Input: part model. Units: mm. Frame: model coordinates. A direction names the side the tool comes from. Round coordinates to 2 decimals unless told otherwise and drop trailing zeros. Loops run counter-clockwise (first coordinate to the right, second up) from the corner with the lowest first, then second, coordinate; pieces in that order, holes last. Notation, with made-up numbers: (46.25, -37.75) -> (67.25, -37.75) arc R9 ccw to (67.25, -27.75) -> close; hole circle Ø1 at (-37.75, -31). An arc over 180 degrees is marked (long way). Answer as a JSON object with one key per item and string values.
```python
from build123d import *

# Parameters (mm, degrees)
F0_R     = 3.175
F1_DEPTH = 25.4
F0_R_2   = 38.1
F2_DEPTH = 12.7
F3_W     = 16.933164
F3_H     = 50.8
F3_W_2   = 16.933333164
F4_DEPTH = 50.8
F5_R     = 25.39999
F6_R     = 3.175
F7_DEPTH = 103.2441
F8_DEPTH = 120.64677


# Not quite as in the source:
# - a fillet or chamfer is up to 0.001 mm smaller than in the source, because OpenCascade refuses the exact size


with BuildPart() as f1:
    # F0 (on Top) → F1 (new body)
    with BuildSketch(Plane.XY):
        Circle(F0_R)
    extrude(amount=-F1_DEPTH)

    # F0 (on Top) → F2 (join)
    with BuildSketch(Plane.XY):
        Circle(F0_R_2)
        Circle(F0_R, mode=Mode.SUBTRACT)
        Circle(F0_R)
    extrude(amount=F2_DEPTH)

    # F3 (on face) → F4 (join)
    with BuildSketch(Plane.XY.offset(12.7)):
        with Locations((16.933418, 0)):
            Rectangle(F3_W, F3_H)
        with Locations((-16.933333418, 0)):
            Rectangle(F3_W_2, F3_H)
    extrude(amount=F4_DEPTH)

    # F5 (radius 25.4 in the source; OpenCascade refuses exactly that, so slightly less here)
    f5_edges = [f1.edges().sort_by_distance(p)[0] for p in [
        (16.933418, -25.4, 63.5),
        (16.933418, 25.4, 63.5),
        (-16.933333, 25.4, 63.5),
        (-16.933333, -25.4, 63.5),
    ]]
    fillet(f5_edges, radius=F5_R)

    # F6 (on face) → F7 (cut)
    with BuildSketch(Plane(origin=(-25.4, 0, 0), x_dir=(0, -1, 0), z_dir=(-1, 0, 0))):
        with Locations((0, 38.1)):
            Circle(F6_R)
    extrude(amount=-F7_DEPTH, mode=Mode.SUBTRACT)

    # F8 (cut): a face of the model
    f8_faces = [f1.faces().sort_by_distance(p)[0] for p in [
        (0, 0, -25.4),
    ]]
    extrude(f8_faces, amount=-F8_DEPTH, mode=Mode.SUBTRACT)


solid = f1.part
```
1) Ray query, probe 1 along X at (y, z) = (16, 14); probe 2 along Z at (x, y) = (13.25, 0) (3 decimals); probe 3 along Y at (x, z) = (0, 4.25) (3 decimals). Return the intervals inside material, ascending.
Output:
{"probe 1": "x = -25.4 to -8.47, 8.47 to 25.4", "probe 2": "z = 0 to 34.925, 41.275 to 63.5", "probe 3": "y = -38.1 to -3.175, 3.175 to 38.1"}
2) Section B-B, the plane z = 54. Output: boundary loops of the cut face in (x, y).
Output:
{"outline": "(-25.4, -19.81) -> (-8.47, -19.81) -> (-8.47, 19.81) -> (-25.4, 19.81) -> close; (8.47, -19.81) -> (25.4, -19.81) -> (25.4, 19.81) -> (8.47, 19.81) -> close"}
3) Contact query for flat-ended pins moving along their axis: P1, Ø4, axis at x = -21.5, z = 45.5, coming from the -Y side; P2, Ø3, axis at x = -10.5, z = 7, coming from the -Y side; P3, Ø2, axis at y = 18.5, z = 17.5, coming from the -X side; P4, Ø5, axis at y = 0, z = 38.1, coming from the +X side. Output: stop coordinate, or through.
Output:
{"P1": "stops at y = -24.82", "P2": "stops at y = -37.02", "P3": "stops at x = -25.4", "P4": "passes through"}
4) Draft query along Z for faces 5 (the face through (25.4, 0, 32)), 6 (the face through (8, 1, 0)), 7 (the face through (17.05, -18.16, 55.86)), 8 (the face through (16.81, 0.69, 35)). Return one class per face: +Z half, -Z half, draft (parallel to the pull), parting line (faces both ways), or undercut.
Output:
{"face 5": "draft", "face 6": "-Z half", "face 7": "+Z half", "face 8": "undercut"}
5) Section D-D, the plane y = -9.5. Output: boundary loops of the cut face in (x, z).
Output:
{"outline": "(-36.9, 0) -> (36.9, 0) -> (36.9, 12.7) -> (25.4, 12.7) -> (25.4, 61.66) -> (8.47, 61.66) -> (8.47, 12.7) -> (-8.47, 12.7) -> (-8.47, 61.66) -> (-25.4, 61.66) -> (-25.4, 12.7) -> (-36.9, 12.7) -> close"}
6) Section C-C, the plane y = 19.5. Output: boundary loops of the cut face in (x, z).
Output:
{"outline": "(-32.73, 0) -> (32.73, 0) -> (32.73, 12.7) -> (25.4, 12.7) -> (25.4, 54.38) -> (8.47, 54.38) -> (8.47, 12.7) -> (-8.47, 12.7) -> (-8.47, 54.38) -> (-25.4, 54.38) -> (-25.4, 12.7) -> (-32.73, 12.7) -> close"}
7) Reachability of faces 1 (the face through (-25.4, 0, 32)), 2 (the face through (-17, -25.4, 25)), 3 (the face through (17, 25.4, 25)), 4 (the face through (8.467, 0, 32)) from +Z, -Z, +X, -X, +Y, -Y: full face, straight path, thin tool, end or side. Return the list, or none.
Output:
{"face 1": "+Z, -X, +Y, -Y", "face 2": "+Z, +X, -X, -Y", "face 3": "+Z, +X, -X, +Y", "face 4": "+Z, +Y, -Y"}
8) Section A-A, the plane x = 0. Output: boundary loops of the cut face in (y, z) (3 decimals), plus the area to 3 significant figures.
Output:
{"outline": "(-38.1, 0) -> (-3.175, 0) -> (-3.175, 12.7) -> (-38.1, 12.7) -> close; (3.175, 0) -> (38.1, 0) -> (38.1, 12.7) -> (3.175, 12.7) -> close", "area": "887 mm^2"}
